The model under review builds one solid part; all positions refer to its coordinate system, in mm. A direction names the side the tool comes from. Round coordinates to 2 decimals unless told otherwise and drop trailing zeros. Write each loop counter-clockwise with the first axis right and the second up, starting at its lowest first coordinate (ties: lowest second). Pieces come first, ordered by that corner, then holes. Notation, with made-up numbers: (-31.75, -18.75) -> (-7.75, -18.75) arc R24 ccw to (-7.75, -3.75) -> close; hole circle Ø8 at (-26, 55). An arc over 180 degrees is marked (long way). Answer in a Markdown table with one row per item. Add a question column.
Autodesk Fusion 360 part; units mm, degrees
sketch "Sketch1" plane through (0, 0, 0) normal (0, 1, 0) x (1, 0, 0)
  circle A0 centre (0, 0) radius 35
  circle A1 centre (0, 0) radius 25
  line L0 (-20, 28.7228) -> (20, 28.7228)
  dimension "d1" = 70
  dimension "d2" = 50
  dimension "d3" = 40
extrude "Extrude1" add sketch "Sketch1" along normal mid plane 15
ref_plane "WorkPlane1" through (0, 0, -50) normal (0, 0, 1) x (1, 0, 0)
sketch "Sketch2" plane through (0, 0, -50) normal (0, 0, 1) x (1, 0, 0)
  line L0 (20, 7.5) -> (-20, 7.5)
  line L1 (-20, 7.5) -> (-20, -7.5)
  line L2 (-20, -7.5) -> (20, -7.5)
  line L3 (20, -7.5) -> (20, 7.5)
  line L4 (20, 7.5) -> (-20, -7.5) construction
  line L5 (-20, 7.5) -> (20, -7.5) construction
  dimension "d7" = 40
  dimension "d8" = 15
extrude "Extrude2" add sketch "Sketch2" along normal blind 23 and the other way blind 100
fillet "Fillet1" radius 20 2 edges at (20, 0, -28.7228) (-20, 0, -28.7228)
fillet "Fillet1" radius 20 2 edges at (20, 0, -150) (-20, 0, -150)
sketch "Sketch3" plane through (0, -7.5, 0) normal (0, -1, 0) x (1, 0, 0)
  circle A0 centre (0, 0) radius 25
  arc A1 (-20, -130) -> (20, -130) centre (0, -130) ccw
  line L0 (20, -130) -> (20, -37.7492)
  arc A2 (25.4545, -24.0222) -> (20, -37.7492) centre (40, -37.7492) ccw
  arc A3 (25.4545, -24.0222) -> (-25.4545, -24.0222) centre (0, 0) ccw
  arc A4 (-20, -37.7492) -> (-25.4545, -24.0222) centre (-40, -37.7492) ccw
  line L1 (-20, -37.7492) -> (-20, -130)
  circle A5 centre (0, -130) radius 5
  dimension "d17" = 10
extrude "Extrude3" cut sketch "Sketch3" against normal through all contours A5
1. Add section A-A on z = 0. Write out the cut boundary in (x, y).
2. For L1, parallel to Z at x = 0, y = 3.25; L2, parallel to X at y = -3.75, z = 0; L3, parallel to Z at x = 3, y = 2.25, list the stretches that pass through material, from the lowest coordinate up.
3. Mouldability with a two-part tool opening along X and no side actions: class faces 1 (the flat face through (20, 0, -85)), 2 (the cylindrical face through (-21.375, -0.105, -30.462)), 3 (the cylindrical face through (23.846, -0.105, 7.509)) as pulls with the +X half, pulls with the -X half, needs draft (parallel to the pull), parting line crosses it, or undercut.
4. Tool access review of faces 4 (the flat face through (-20, 0, -85)), 5 (the flat face through (0, 7.5, -79)): name each direction out of +Z, -Z, +X, -X, +Y, -Y from which nothing blocks a thin tool from reaching the whole face with its end or side.
5. Add section D-D on z = -115.5. Write out the cut boundary in (x, y).
6. Insertion check: pin 1 Ø4.5 at (y, z) = (-1, -75) entering from -X; pin 2 Ø3 at (x, y) = (20, -1) entering from -Z; pin 3 Ø5 at (x, y) = (-26.5, 3.5) entering from -Z. Each pin has a flat end and moves straight along its axis. Give the tip position at first contact, or say it passes through.
7. Add section B-B on y = 0.75. State how many separate pieces and enclosed holes the cut face has, plus the area to 3 significant figures.
8. Add section C-C on x = -12. Write out the cut boundary in (y, z).
Filled in:
| question | item | result |
|---|---|---|
| 1 | outline | (-35, -7.5) -> (-25, -7.5) -> (-25, 7.5) -> (-35, 7.5) -> close; (25, -7.5) -> (35, -7.5) -> (35, 7.5) -> (25, 7.5) -> close |
| 2 | L1 | -150 to -135, -125 to -25, 25 to 35 |
| 2 | L2 | -35 to -25, 25 to 35 |
| 2 | L3 | -149.77 to -134, -126 to -24.82, 24.82 to 34.87 |
| 3 | face 1 | pulls with the +X half |
| 3 | face 2 | pulls with the -X half |
| 3 | face 3 | undercut |
| 4 | face 4 | -Z, -X, +Y, -Y |
| 4 | face 5 | +Z, -Z, +X, -X, +Y |
| 5 | outline | (-20, -7.5) -> (20, -7.5) -> (20, 7.5) -> (-20, 7.5) -> close |
| 6 | pin 1 | x = -20 |
| 6 | pin 2 | z = -137.6 |
| 6 | pin 3 | z = -25.75 |
| 7 | separate pieces | 1 |
| 7 | enclosed holes | 2 |
| 7 | area | 6,330 mm² |
| 8 | outline | (-7.5, -146) -> (7.5, -146) -> (7.5, -21.93) -> (-7.5, -21.93) -> close; (-7.5, 21.93) -> (7.5, 21.93) -> (7.5, 32.88) -> (-7.5, 32.88) -> close |
